Work out the finished part from the listing and answer in its coordinate system (mm). A direction names the side the tool comes from. Give positions to 0.01 mm unless a question says otherwise; leave off trailing zeros. Order: outer loops, then holes, each group sorted by start corner. A loop starts at its lowest first (then second) coordinate and runs counter-clockwise, first axis right, second up.
```python
from build123d import *

# Parameters (mm, degrees)
SKETCH_1_W          = 41
SKETCH_1_H          = 41
EXTRUDE_1_DEPTH     = 11.8
CHAMFER_1_SIZE      = 3
FILLET_1_R          = 5
SKETCH_3_R          = 16.5
CUT_EXTRUDE_2_DEPTH = 3
SKETCH_4_R          = 5
CUT_EXTRUDE_3_DEPTH = 31.297524651
SKETCH_5_W          = 30
SKETCH_5_H          = 6
CUT_EXTRUDE_4_DEPTH = 3
CHAMFER_2_SIZE      = 1.6
SKETCH_6_R          = 14.25
CUT_EXTRUDE_5_DEPTH = 2
CUT_EXTRUDE_6_DEPTH = 1
SKETCH_8_R          = 1.6
CUT_EXTRUDE_7_DEPTH = 32.300798712
SKETCH_9_R          = 3.75
CUT_EXTRUDE_8_DEPTH = 4


with BuildPart() as part:
    # ｽｹｯﾁ1 → ﾎﾞｽ - 押し出し1 (new body)
    with BuildSketch(Plane.XY):
        Rectangle(SKETCH_1_W, SKETCH_1_H)
    extrude(amount=EXTRUDE_1_DEPTH)

    # 面取り1
    chamfer_1_edges = [part.edges().sort_by_distance(p)[0] for p in [
        (-20.5, 0, 11.8),
        (0, -20.5, 11.8),
        (20.5, 0, 11.8),
        (0, 20.5, 11.8),
    ]]
    chamfer(chamfer_1_edges, length=CHAMFER_1_SIZE)

    # ﾌｨﾚｯﾄ1
    # the kernel refuses this fillet: 5 mm, written as the material it takes off along each edge
    with BuildSketch(Plane(origin=(20.5, -20.5, -12.5), x_dir=(-1, 0, 0), z_dir=(0, 0, 1)), Plane(origin=(20.5, 20.5, -12.5), x_dir=(0, -1, 0), z_dir=(0, 0, 1))) as fillet_1_piece_1:
        with BuildLine():
            CenterArc((FILLET_1_R, -FILLET_1_R), FILLET_1_R, 90, 90)
            Line((0, -FILLET_1_R), (0, 0))
            Line((0, 0), (FILLET_1_R, 0))
        make_face()
    extrude(amount=33.8, mode=Mode.SUBTRACT)
    with BuildSketch(Plane(origin=(-20.5, -20.5, -12.5), x_dir=(1, 0, 0), z_dir=(0, 0, 1)), Plane(origin=(-20.5, 20.5, -12.5), x_dir=(0, -1, 0), z_dir=(0, 0, 1))) as fillet_1_piece_2:
        with BuildLine():
            CenterArc((FILLET_1_R, FILLET_1_R), FILLET_1_R, 180, 90)
            Line((0, FILLET_1_R), (0, 0))
            Line((0, 0), (FILLET_1_R, 0))
        make_face()
    extrude(amount=33.8, mode=Mode.SUBTRACT)
    with BuildSketch(Plane(origin=(-24.666666667, 24.666666667, 4.633333333), x_dir=(-0.408248290463863, -0.816496580927726, -0.408248290463863), z_dir=(0.5773502691896258, -0.5773502691896258, 0.5773502691896258)), Plane(origin=(-24.666666667, -24.666666667, 4.633333333), x_dir=(0.816496580927726, -0.408248290463863, -0.408248290463863), z_dir=(0.5773502691896258, 0.5773502691896258, 0.5773502691896258))) as fillet_1_piece_3:
        with BuildLine():
            CenterArc((FILLET_1_R * 0.57735026919, FILLET_1_R), FILLET_1_R, 210, 60)
            Line((-FILLET_1_R * 0.288675134595, FILLET_1_R * 0.5), (0, 0))
            Line((0, 0), (FILLET_1_R * 0.57735026919, 0))
        make_face()
    extrude(amount=19.629909152, mode=Mode.SUBTRACT)
    with BuildSketch(Plane(origin=(24.666666667, 24.666666667, 4.633333333), x_dir=(0.40824829046386313, -0.816496580927726, -0.40824829046386285), z_dir=(-0.5773502691896258, -0.5773502691896258, 0.5773502691896258)), Plane(origin=(24.666666667, -24.666666667, 4.633333333), x_dir=(-0.816496580927726, -0.40824829046386285, -0.4082482904638632), z_dir=(-0.5773502691896258, 0.5773502691896258, 0.5773502691896258))) as fillet_1_piece_4:
        with BuildLine():
            CenterArc((FILLET_1_R * 0.57735026919, -FILLET_1_R), FILLET_1_R, 90, 60)
            Line((-FILLET_1_R * 0.288675134595, -FILLET_1_R * 0.5), (0, 0))
            Line((0, 0), (FILLET_1_R * 0.57735026919, 0))
        make_face()
    extrude(amount=19.629909152, mode=Mode.SUBTRACT)

    # ｽｹｯﾁ3 → ｶｯﾄ - 押し出し2 (cut)
    with BuildSketch(Plane(origin=(0, 0, 0), x_dir=(-1, 0, 0), z_dir=(0, 0, -1))):
        Circle(SKETCH_3_R)
    extrude(amount=-CUT_EXTRUDE_2_DEPTH, mode=Mode.SUBTRACT)

    # ｽｹｯﾁ4 → ｶｯﾄ - 押し出し3 (cut, through all)
    with BuildSketch(Plane(origin=(0, 0, 3), x_dir=(-1, 0, 0), z_dir=(0, 0, -1))):
        Circle(SKETCH_4_R)
    extrude(amount=-CUT_EXTRUDE_3_DEPTH, mode=Mode.SUBTRACT)

    # ｽｹｯﾁ5 → ｶｯﾄ - 押し出し4 (cut)
    with BuildSketch(Plane(origin=(0, 0, 0), x_dir=(-1, 0, 0), z_dir=(0, 0, -1))):
        with Locations((0, 15.2)):
            Rectangle(SKETCH_5_W, SKETCH_5_H)
        with Locations((0, -15.2)):
            Rectangle(SKETCH_5_W, SKETCH_5_H)
    extrude(amount=-CUT_EXTRUDE_4_DEPTH, mode=Mode.SUBTRACT)

    # 面取り2
    chamfer_2_edges = [part.edges().sort_by_distance(p)[0] for p in [
        (5, 0, 3),
    ]]
    chamfer(chamfer_2_edges, length=CHAMFER_2_SIZE)

    # ｽｹｯﾁ6 → ｶｯﾄ - 押し出し5 (cut)
    with BuildSketch(Plane.XY.offset(11.8)):
        Circle(SKETCH_6_R)
    extrude(amount=-CUT_EXTRUDE_5_DEPTH, mode=Mode.SUBTRACT)

    # ｽｹｯﾁ7 → ｶｯﾄ - 押し出し6 (cut)
    with BuildSketch(Plane(origin=(0, -14.65, 14.65), x_dir=(1, 0, 0), z_dir=(0, -0.7071067811865491, 0.707106781186546))):
        Polygon((0, -7.77314934), (1.812279996, -4.634188309), (-1.812279996, -4.634188309), align=None)
    extrude(amount=-CUT_EXTRUDE_6_DEPTH, mode=Mode.SUBTRACT)

    # ｽｹｯﾁ8 → ｶｯﾄ - 押し出し7 (cut, through all)
    with BuildSketch(Plane.XY.offset(11.8)):
        with Locations((-17, 17)):
            Circle(SKETCH_8_R)
        with Locations((-17, -17)):
            Circle(SKETCH_8_R)
        with Locations((17, -17)):
            Circle(SKETCH_8_R)
        with Locations((17, 17)):
            Circle(SKETCH_8_R)
    extrude(amount=-CUT_EXTRUDE_7_DEPTH, mode=Mode.SUBTRACT)

    # ｽｹｯﾁ9 → ｶｯﾄ - 押し出し8 (cut)
    with BuildSketch(Plane.XY.offset(11.8)):
        with Locations((17, 17)):
            Circle(SKETCH_9_R)
        with Locations((-17, 17)):
            Circle(SKETCH_9_R)
        with Locations((-17, -17)):
            Circle(SKETCH_9_R)
        with Locations((17, -17)):
            Circle(SKETCH_9_R)
    extrude(amount=-CUT_EXTRUDE_8_DEPTH, mode=Mode.SUBTRACT)


solid = part.part
```
1. The part is cut by section C-C (x = 17). Write down the section's boundary in (y, z).
Findings below:
outline: (-20.27, 0) - (-18.6, 0) - (-18.6, 7.8) - (-20.27, 7.8) - close; (-15.4, 0) - (15.4, 0) - (15.4, 7.8) - (13.25, 7.8) - (13.25, 11.8) - (-13.25, 11.8) - (-13.25, 7.8) - (-15.4, 7.8) - close; (18.6, 0) - (20.27, 0) - (20.27, 7.8) - (18.6, 7.8) - close
2. The part is cut by section B-B (z = 1.75). Write down the section's boundary in (x, y), then the cut area to 3 significant figures.
Findings below:
outline: (-20.5, -15.5) arc R5 ccw to (-15.5, -20.5) - (15.5, -20.5) arc R5 ccw to (20.5, -15.5) - (20.5, 15.5) arc R5 ccw to (15.5, 20.5) - (-15.5, 20.5) arc R5 ccw to (-20.5, 15.5) - close; hole circle Ø3.2 at (-17, -17); hole circle Ø3.2 at (-17, 17); hole (-15, -18.2) - (15, -18.2) - (15, -12.2) - (11.11, -12.2) arc R16.5 ccw to (11.11, 12.2) - (15, 12.2) - (15, 18.2) - (-15, 18.2) - (-15, 12.2) - (-11.11, 12.2) arc R16.5 ccw to (-11.11, -12.2) - (-15, -12.2) - close; hole circle Ø3.2 at (17, -17); hole circle Ø3.2 at (17, 17)
area: 543 mm2
3. The mould has two halves that part along Y. Classify faces 1 (the face through (19, -0.2, 10.3)), 2 (the face through (13, -12.2, 1)), 3 (the face through (-19, 19.07, 3.36)): pulls with the +Y half, pulls with the -Y half, needs draft (parallel to the pull), parting line crosses it, or undercut.
Findings below:
face 1: needs draft
face 2: undercut
face 3: pulls with the +Y half
4. Given P1, Ø3.5, axis at x = -18, y = -18, coming from the +Z side; P2, Ø5, axis at x = -2, y = -5, coming from the +Z side; P3, Ø2.5, axis at x = 17, y = 17, coming from the +Z side, each flat-ended and moving along its own axis, determine where each tip first touches the part or whether it passes through.
Findings below:
P1: stops at z = 7.8
P2: stops at z = 9.8
P3: passes through
5. Straight lines are drawn through the part: probe 1 along Y at (x, z) = (-17, 3.25); probe 2 along Y at (x, z) = (5, 1.5); probe 3 along Y at (x, z) = (-15, 8.5). For each, find the intervals that lie inside material, in ascending order.
Findings below:
probe 1: y = -20.27 to -18.6, -15.4 to 15.4, 18.6 to 20.27
probe 2: y = -20.5 to -18.2, 18.2 to 20.5
probe 3: y = -20.5 to -20.17, -13.83 to 13.83, 20.17 to 20.5
6. The part is cut by section D-D (y = 17). Write down the section's boundary in (x, z), then the cut area to 3 significant figures.
Findings below:
outline: (-20.27, 0) - (-18.6, 0) - (-18.6, 7.8) - (-20.27, 7.8) - close; (-15.4, 0) - (-15, 0) - (-15, 3) - (15, 3) - (15, 0) - (15.4, 0) - (15.4, 7.8) - (13.25, 7.8) - (13.25, 11.8) - (-13.25, 11.8) - (-13.25, 7.8) - (-15.4, 7.8) - close; (18.6, 0) - (20.27, 0) - (20.27, 7.8) - (18.6, 7.8) - close
area: 282 mm2
7. Which of the six approach directions +Z, -Z, +X, -X, +Y, -Y give full straight-line access (tool end or side, diameter ignored) to faces 4 (the face through (0.893, -18.704, 9.899)), 5 (the face through (16.5, 0.2, 1.5)), 6 (the face through (15, -17, 7.8)), 7 (the face through (-8, 12, 11.8))?
Findings below:
face 4: none
face 5: -Z
face 6: +Z
face 7: +Z, +X, -X, +Y, -Y
8. The part is cut by section A-A (y = 0). Write down the section's boundary in (x, z), then the cut area to 3 significant figures.
Findings below:
outline: (-20.5, 0) - (-16.5, 0) - (-16.5, 3) - (-6.6, 3) - (-5, 4.6) - (-5, 9.8) - (-14.25, 9.8) - (-14.25, 11.8) - (-17.5, 11.8) - (-20.5, 8.8) - close; (5, 4.6) - (6.6, 3) - (16.5, 3) - (16.5, 0) - (20.5, 0) - (20.5, 8.8) - (17.5, 11.8) - (14.25, 11.8) - (14.25, 9.8) - (5, 9.8) - close
area: 248 mm2
